Source: CAD feature listing. Evaluate the final solid. Frame: model axes, mm. A direction names the side the tool comes from. Round coordinates to 2 decimals unless told otherwise and drop trailing zeros. Order: outer loops, then holes, each group sorted by start corner. A loop starts at its lowest first (then second) coordinate and runs counter-clockwise, first axis right, second up. Notation, with made-up numbers: (-30, -38.5) - (3, -38.5) arc R10 ccw to (3, -34.5) - close; hole circle Ø1 at (22.25, -31). An arc over 180 degrees is marked (long way). Put each result on its own line as item: value. Start each with the question number.
1) Line query: probe 1 along Z at (x, y) = (130, -53.5); probe 2 along Z at (x, y) = (24, -125); probe 3 along Z at (x, y) = (179, -16.5). Output: solid intervals per line, ascending. Write a range as [from, to].
2) Section B-B on x = 50. Output: boundary loops of the cut face in (y, z), then the cut area to 3 significant figures.
3) Section C-C on z = 67. Output: boundary loops of the cut face in (x, y), then the cut area to 3 significant figures.
4) Access query for faces 1 (the face through (192.69, -123.25, 40.15)), 2 (the face through (110, -123, 82.151)). Directions: +Z, -Z, +X, -X, +Y, -Y. A direction counts if a zero-diameter tool reaches every point of the face in a straight line with its end or side. Return the directions, or none.
5) Section A-A on y = -135.5. Output: boundary loops of the cut face in (x, z).
6) Contact query for flat-ended pins moving along their axis: P1, Ø8, axis at y = -114, z = 37, coming from the +X side; P2, Ø0.5, axis at y = -67.5, z = 82.5, coming from the -X side. Output: stop coordinate, or through.
7) Mould query, pull axis Z, two halves, no side actions, for faces 3 (the face through (36, -123, -1)), 4 (the face through (191.69, -123.25, 41.98)), 5 (the face through (110, -123, 83.151)). Classes: +Z half, -Z half, draft (parallel to the pull), parting line (faces both ways), or undercut.
```python
from build123d import *

# Parameters (mm, degrees)
F1_DEPTH  = 250
F1_FACE_W = 250
F1_FACE_H = 1
F2_DEPTH  = 25


with BuildPart() as f1:
    # F0 (on Front) → F1 (new body)
    with BuildSketch(Plane.XZ):
        with BuildLine():
            Line((150.622934, 0), (-75.805686, 0))
            Line((-75.805686, 0), (-75.805686, -1))
            Line((-75.805686, -1), (150.622934, -1))
            ThreePointArc((150.622934, -1), (192.698204, 41.07527), (150.622934, 83.15054))
            Line((150.622934, 83.15054), (92.919543, 83.15054))
            Line((92.919543, 83.15054), (92.919543, 82.15054))
            Line((92.919543, 82.15054), (150.622934, 82.15054))
            ThreePointArc((150.622934, 82.15054), (191.698204, 41.07527), (150.622934, 0))
        make_face()
    extrude(amount=F1_DEPTH)

    # F1_face (on face) → F2 (join)
    with BuildSketch(Plane(origin=(92.919543, -125, 82.65054), x_dir=(0, -1, 0), z_dir=(-1, 0, 0))):
        Rectangle(F1_FACE_W, F1_FACE_H)
    extrude(amount=F2_DEPTH)


solid = f1.part
```
Answer sheet:
1. probe 1: [-1, 0], [82.15, 83.15]
1. probe 2: [-1, 0]
1. probe 3: [10.01, 11.38], [70.77, 72.14]
2. outline: (-250, -1) - (0, -1) - (0, 0) - (-250, 0) - close
2. area: 250 mm^2
3. outline: (182.48, -250) - (183.76, -250) - (183.76, 0) - (182.48, 0) - close
3. area: 320 mm^2
4. face 1: +X, +Y, -Y
4. face 2: -X, +Y, -Y
5. outline: (-75.81, -1) - (150.62, -1) arc R42.08 ccw to (150.62, 83.15) - (67.92, 83.15) - (67.92, 82.15) - (150.62, 82.15) arc R41.08 cw to (150.62, 0) - (-75.81, 0) - close
6. P1: x = 192.7
6. P2: x = 67.92
7. face 3: -Z half
7. face 4: undercut
7. face 5: +Z half
